```python
from build123d import *

# Parameters (mm, degrees)
SKETCH2_W           = 31.75
SKETCH2_H           = 12.7
REVOLVE1_ANGLE      = 180
SKETCH3_R           = 5.08
BOSS_EXTRUDE1_DEPTH = 62.23
SKETCH4_W           = 19.5326
SKETCH4_H           = 6.35
BOSS_EXTRUDE2_DEPTH = 76.2
SKETCH5_R           = 8.89
CUT_EXTRUDE1_DEPTH  = 76.2


with BuildPart() as part:
    # Sketch2 → Revolve1 (revolve)
    with BuildSketch(Plane.XY):
        with Locations((15.875, 6.35)):
            Rectangle(SKETCH2_W, SKETCH2_H)
    revolve(axis=Axis((31.75, 0, 0), (0, 1, 0)), revolution_arc=REVOLVE1_ANGLE)

    # Sketch3 → Boss-Extrude1 (add)
    with BuildSketch(Plane(origin=(0, 0, 0), x_dir=(-1, 0, 0), z_dir=(0, 0, -1))):
        with Locations((-47.625, 6.35)):
            Circle(SKETCH3_R)
        with Locations((-15.875, 6.35)):
            Circle(SKETCH3_R)
    extrude(amount=BOSS_EXTRUDE1_DEPTH)

    # Sketch4 → Boss-Extrude2 (add)
    with BuildSketch(Plane(origin=(0, 0, 0), x_dir=(-1, 0, 0), z_dir=(0, 0, -1))):
        with Locations((-31.7373, 3.175)):
            Rectangle(SKETCH4_W, SKETCH4_H)
    extrude(amount=BOSS_EXTRUDE2_DEPTH)

    # Sketch5 → Cut-Extrude1 (cut)
    with BuildSketch(Plane(origin=(0, 6.35, 0), x_dir=(1, 0, 0), z_dir=(0, 1, 0))):
        with Locations((31.75, 27.94)):
            Circle(SKETCH5_R)
    extrude(amount=-CUT_EXTRUDE1_DEPTH, mode=Mode.SUBTRACT)


solid = part.part
```
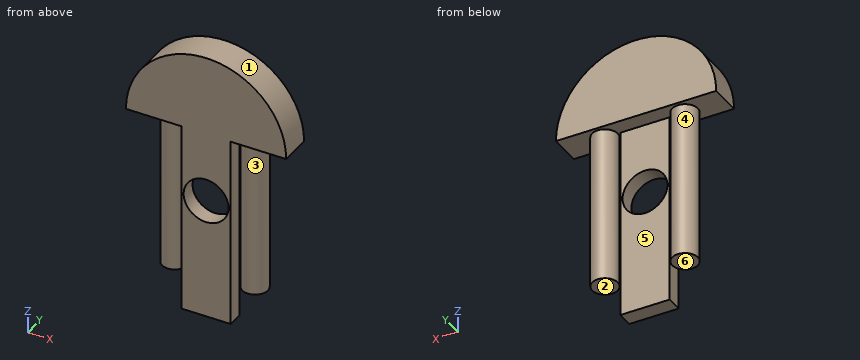
Here's how the part is built. I have some questions about the finished solid (model axes, mm). Face numbers are marked on the shaded views. A direction names the side the tool comes from. Give positions to 0.01 mm unless a question says otherwise; leave off trailing zeros. Loops run counter-clockwise (first coordinate to the right, second up) from the corner with the lowest first, then second, coordinate; pieces in that order, holes last. Notation, with made-up numbers: M -34.75,41 L -17.75,41 A16 cw -17.75,67 Z; hole C -28,28.5 d10. An arc over 180 degrees is marked long. Put each result on its own line as item: value. Start each with the question number.
(1) I need wall thicknesses on line 1 along Z through (x, y) = (31.75, 2.75); line 2 along X through (y, z) = (4, -27.94); line 3 along X through (y, z) = (3.5, -27.94). Which ranges of each line are inside material? Lowest first, please. Write a range as [from, to].
(2) Will these pins go through, and if not, where does the flat tip stop? pin 1 Ø5 at (x, y) = (37.5, 6) entering from +Z; pin 2 Ø7 at (y, z) = (4, -38.5) entering from -X (3 decimals); pin 3 Ø1.9 at (y, z) = (3, -47.5) entering from +X.
(3) I want a section at B-B on z = -27.94. Please give me the cut outline in (x, y) (3 decimals).
(4) I want a section at D-D on y = 4.25. Please give me the cut outline in (x, z).
(5) I want a section at A-A on x = 31.75. Please give me the cut outline in (y, z).
(6) If we mould it in two halves opening along X, with no side actions, what happens to the marked faces 1, 2 and 3? For each: +X half, -X half, draft (parallel to the pull), parting line (faces both ways), or undercut.
(7) For the marked faces 4, 5 and 6, which set-ups out of +Z, -Z, +X, -X, +Y, -Y let a thin tool reach every point of the face, with its end or its side?
(8) I want a section at C-C on z = -12.5. Please give me the cut outline in (x, y) (3 decimals).
Answer block:
1. line 1: [-76.2, -36.83], [-19.05, 31.75]
1. line 2: [11.37, 20.38], [21.97, 22.86], [40.64, 41.5], [43.12, 52.13]
1. line 3: [11.67, 20.08], [21.97, 22.86], [40.64, 41.5], [43.42, 51.83]
2. pin 1: z = 31.58
2. pin 2: x = 10.795
2. pin 3: x = 52.1
3. outline: C 15.875,6.35 d10.16; M 21.971,0 L 22.86,0 L 22.86,6.35 L 21.971,6.35 Z; M 40.64,0 L 41.504,0 L 41.504,6.35 L 40.64,6.35 Z; C 47.625,6.35 d10.16
4. outline: M 0,0 L 11.25,0 L 11.25,-62.23 L 20.5,-62.23 L 20.5,0 L 21.97,0 L 21.97,-76.2 L 41.5,-76.2 L 41.5,0 L 43,0 L 43,-62.23 L 52.25,-62.23 L 52.25,0 L 63.5,0 A31.75 ccw Z; hole C 31.75,-27.94 d17.78
5. outline: M 0,-76.2 L 6.35,-76.2 L 6.35,-36.83 L 0,-36.83 Z; M 0,-19.05 L 6.35,-19.05 L 6.35,0 L 12.7,0 L 12.7,31.75 L 0,31.75 Z
6. face 1: parting line
6. face 2: draft
6. face 3: undercut
7. face 4: -Z
7. face 5: -Z, +Y
7. face 6: -Z, -X, +Y, -Y
8. outline: C 15.875,6.35 d10.16; M 21.971,0 L 41.504,0 L 41.504,6.35 L 21.971,6.35 Z; C 47.625,6.35 d10.16
